Geometry: see drawing. Coordinates: mm, zero at the bounding-box minimum. A direction names the side the tool comes from. Give positions to 0.01 mm unless a question says otherwise; leave off trailing zeros. Write each loop counter-clockwise with the first axis right and the second up, starting at its lowest first coordinate (ties: lowest second). Pieces come first, ordered by that corner, then holes. Notation, with made-up numbers: M -30.75,-38 L 7.25,-38 A13 cw 7.25,-19 Z; hole C -16,54.25 d2. An arc over 180 degrees is marked long. Use one line per item in the form item = value. Start each with the question number.
Item 1: Pull-direction query (Y, two-part tool) for the marked faces 5, 6 and 7; classes: released by +Y, released by -Y, zero draft, split by the parting line, or undercut.
Item 2: Access query for the marked faces 1, 2, 3 and 4. Directions: +Z, -Z, +X, -X, +Y, -Y. A direction counts if a zero-diameter tool reaches every point of the face in a straight line with its end or side. Return the directions, or none.
Item 3: Contact query for flat-ended pins moving along their axis: P1, Ø8, axis at y = 63, z = 17, coming from the -X side; P2, Ø8, axis at x = 4, y = 55, coming from the -Z side; P3, Ø1.8, axis at x = 7, z = 4, coming from the -Y side. Output: stop coordinate, or through.
Item 4: Material intervals for line 1 along Z through (x, y) = (17.75, 38); line 2 along Y through (x, z) = (14, 16.25); line 3 along X through (y, z) = (50, 9) (1 decimal), sorted ascending. Write a range as from..to.
Item 5: Section query D-D on y = 14.5. Return loops of the section in (x, z) (1 decimal), then the cut area to 3 significant figures.
Item 6: Section query B-B on x = 10. Return loops of the section in (y, z).
Item 7: Section query A-A on z = 10. Return loops of the section in (x, y) (1 decimal), then the cut area to 3 significant figures.
Item 8: Section query C-C on y = 66.5. Return loops of the section in (x, z).
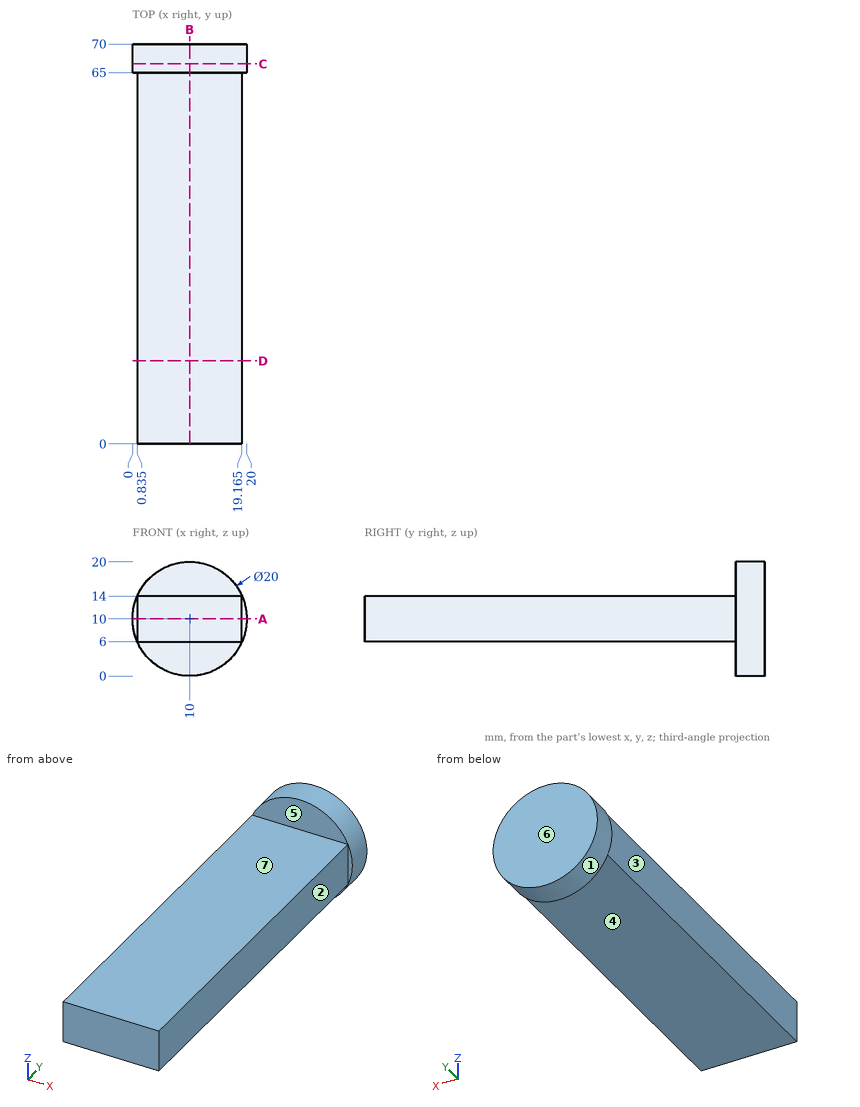
Answer sheet:
q1.face_5 = released by -Y
q1.face_6 = released by +Y
q1.face_7 = zero draft
q2.face_1 = +Y, -Y
q2.face_2 = +Z, -Z, +X, -Y
q2.face_3 = +Z, -Z, -X, -Y
q2.face_4 = -Z, +X, -X, -Y
q3.P1 = 0.65
q3.P2 = 6
q3.P3 = 65
q4.line_1 = 6..14
q4.line_2 = 65..70
q4.line_3 = 0.8..19.2
q5.outline = M 0.8,6 L 19.2,6 L 19.2,14 L 0.8,14 Z
q5.area = 147 mm2
q6.outline = M 0,6 L 65,6 L 65,0 L 70,0 L 70,20 L 65,20 L 65,14 L 0,14 Z
q7.outline = M 0,65 L 0.8,65 L 0.8,0 L 19.2,0 L 19.2,65 L 20,65 L 20,70 L 0,70 Z
q7.area = 1,290 mm2
q8.outline = C 10,10 d20
